```python
from build123d import *

# Parameters (mm, degrees)
ESQUISSE1_W             = 30
ESQUISSE1_H             = 71
BOSS_EXTRU_1_DEPTH      = 6
ESQUISSE3_R             = 1.85
ESQUISSE3_W             = 10
ESQUISSE3_H             = 6
ENL_V_MAT_EXTRU_1_DEPTH = 6


with BuildPart() as part:
    # Esquisse1 → Boss.-Extru.1 (new body)
    with BuildSketch(Plane.XY):
        with Locations((-15, 35.5)):
            Rectangle(ESQUISSE1_W, ESQUISSE1_H)
    extrude(amount=BOSS_EXTRU_1_DEPTH)

    # Esquisse3 → Enlèv. mat.-Extru.1 (cut)
    with BuildSketch(Plane(origin=(0, 0, 0), x_dir=(-1, 0, 0), z_dir=(0, 0, -1))):
        with Locations((4.8, 66.4)):
            Circle(ESQUISSE3_R)
        with Locations((25.2, 66.4)):
            Circle(ESQUISSE3_R)
        with Locations((5, 3)):
            Rectangle(ESQUISSE3_W, ESQUISSE3_H)
        with Locations((25, 3)):
            Rectangle(ESQUISSE3_W, ESQUISSE3_H)
    extrude(amount=-ENL_V_MAT_EXTRU_1_DEPTH, mode=Mode.SUBTRACT)


solid = part.part
```
Could you check a few things on this model? Use its own coordinates, in mm. A direction names the side the tool comes from. Round coordinates to 2 decimals unless told otherwise and drop trailing zeros. Loops run counter-clockwise (first coordinate to the right, second up) from the corner with the lowest first, then second, coordinate; pieces in that order, holes last. Notation, with made-up numbers: M 27,-34 L 80,-34 A24 ccw 80,0 Z; hole C 1.5,79 d11. An arc over 180 degrees is marked long. Put each result on its own line as item: value.
Q1. On a 3-axis mill with a long thin cutter (end or side, diameter ignored), from which of +Z, -Z, +X, -X, +Y, -Y can I reach the whole of each face in a straight line? I mean faces 5 (the face through (-20, 3, 3)), 6 (the face through (-30, 38, 3)), 7 (the face through (-10, 3, 3)). Say none if no direction works.
Check result:
face 5: +Z, -Z, -X, -Y
face 6: +Z, -Z, -X, +Y, -Y
face 7: +Z, -Z, +X, -Y
Q2. Imagine slicing it at C-C (z = 3.05). Write out the boundary of the cut face in (x, y), then the cut area to 3 significant figures.
Check result:
outline: M -30,6 L -20,6 L -20,0 L -10,0 L -10,6 L 0,6 L 0,71 L -30,71 Z; hole C -25.2,66.4 d3.7; hole C -4.8,66.4 d3.7
area: 1,990 mm2
Q3. Thinking about a two-plate mould opening in Y: for faces 1 (the face through (-15, 36, 0)), 2 (the face through (-4.559, 68.234, 2.958)), 3 (the face through (-25, 6, 3)), 4 (the face through (-23.836, 67.65, 2.958)), which applies, released by +Y, released by -Y, zero draft, split by the parting line, or undercut?
Check result:
face 1: zero draft
face 2: undercut
face 3: released by -Y
face 4: undercut
Q4. I need wall thicknesses on probe 1 along X at (y, z) = (66.4, 3.4); probe 2 along Y at (x, z) = (-4.8, 2.35); probe 3 along Y at (x, z) = (-9.5, 0.8). Which ranges of each line are inside material? Lowest first, please.
Check result:
probe 1: -30 to -27.05, -23.35 to -6.65, -2.95 to 0
probe 2: 6 to 64.55, 68.25 to 71
probe 3: 6 to 71
Q5. Imagine slicing it at B-B (y = 66.4). Write out the boundary of the cut face in (x, z), then the cut area to 3 significant figures.
Check result:
outline: M -30,0 L -27.05,0 L -27.05,6 L -30,6 Z; M -23.35,0 L -6.65,0 L -6.65,6 L -23.35,6 Z; M -2.95,0 L 0,0 L 0,6 L -2.95,6 Z
area: 136 mm2
Q6. For pin 1 (3 mm diameter, centred on y = 4, z = 3.5, fed in from -X); pin 2 (1.8 mm diameter, centred on x = -4.5, z = 2.5, fed in from -Y); pin 3 (2 mm diameter, centred on x = -25.2, y = 66.4, fed in from -Z), each with a flat end and sliding along its axis, tell me the tip position at first contact or that it passes through.
Check result:
pin 1: x = -20
pin 2: y = 6
pin 3: through
Q7. Imagine slicing it at A-A (x = -25.2). Write out the boundary of the cut face in (y, z), then the cut area to 3 significant figures.
Check result:
outline: M 6,0 L 64.55,0 L 64.55,6 L 6,6 Z; M 68.25,0 L 71,0 L 71,6 L 68.25,6 Z
area: 368 mm2
